Here's how the part is built. I have some questions about the finished solid (model axes, mm). Round coordinates to 2 decimals unless told otherwise and drop trailing zeros. Loops run counter-clockwise (first coordinate to the right, second up) from the corner with the lowest first, then second, coordinate; pieces in that order, holes last. Notation, with made-up numbers: M -30,-9.75 L 23,-9.75 A21 cw 23,9.25 Z; hole C 25.25,57 d11. An arc over 180 degrees is marked long. Put each result on its own line as item: value. Start each with the question number.
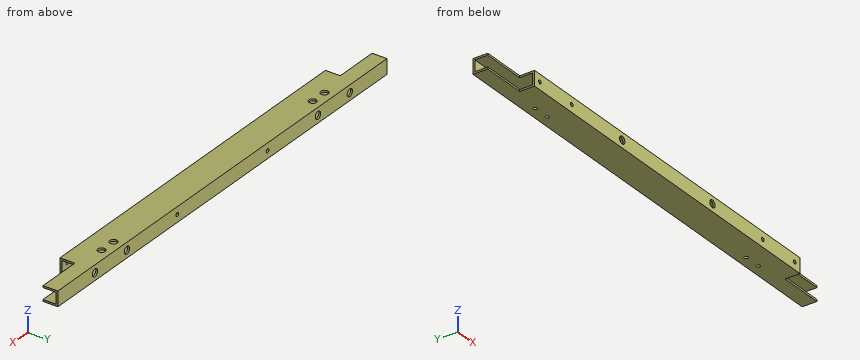
Autodesk Inventor part; units mm, degrees
ref_plane "YZ Plane" through (0, 0, 0) normal (1, 0, 0) x (0, 1, 0)
ref_plane "XZ Plane" through (0, 0, 0) normal (0, 1, 0) x (-1, 0, 0)
ref_plane "XY Plane" through (0, 0, 0) normal (0, 0, 1) x (1, 0, 0)
sketch "Sketch1" plane through (0, 0, 0) normal (0, 0, 1) x (1, 0, 0)
  line L0 (0, 0) -> (787.4, 0)
  line L1 (787.4, 0) -> (787.4, 50.8)
  line L2 (787.4, 50.8) -> (565.5048, 50.8)
  line L3 (565.5048, 50.8) -> (348.1028, 50.8)
  line L4 (348.1028, 50.8) -> (130.7008, 50.8)
  line L5 (130.7008, 50.8) -> (0, 50.8)
  line L6 (0, 50.8) -> (0, 0)
  dimension "d2" = 50.8
  dimension "d3" = 50.8
  dimension "d4" = 787.4
extrude "Extrusion1" add sketch "Sketch1" along normal blind 25.4
shell "Shell1" thickness 3.175 removed faces 2 at (0, 33.8667, 16.9333) at (787.4, 16.9333, 16.9333)
sketch "Sketch2" plane through (0, 0, 25.4) normal (0, 0, 1) x (1, 0, 0)
  line L0 (0, 0) -> (76.2, 0)
  line L1 (76.2, 0) -> (76.2, 25.4)
  line L2 (76.2, 25.4) -> (0, 25.4)
  line L3 (0, 25.4) -> (0, 0)
  line L4 (787.4, 0) -> (711.2, 0)
  line L5 (711.2, 0) -> (711.2, 25.4)
  line L6 (711.2, 25.4) -> (787.4, 25.4)
  line L7 (787.4, 25.4) -> (787.4, 0)
  dimension "d9" = 25.4
  dimension "d12" = 76.2
extrude "Extrusion2" cut sketch "Sketch2" against normal through all
sketch "Sketch4" plane through (0, 50.8, 0) normal (0, 1, 0) x (1, 0, 0)
  line L0 (787.4, 0) -> (787.4, -25.4)
  line L1 (787.4, 0) -> (0, 0)
  circle A0 centre (501.65, -12.7) radius 3.175
  circle A1 centre (285.75, -12.7) radius 3.175
  dimension "d21" = 285.75
  dimension "d22" = 215.9
  dimension "d23" = 12.7
  dimension "d24" = 12.7
  dimension "d25" = 6.35
  dimension "d26" = 6.35
extrude "Extrusion4" cut sketch "Sketch4" against normal through all
sketch "Sketch5" plane through (76.2, 0, 0) normal (0, -1, 0) x (1, 0, 0)
  circle A0 centre (209.55, 12.7) radius 3.175
  circle A1 centre (425.45, 12.7) radius 3.175
  circle A2 centre (209.55, 12.7) radius 6.35
  circle A3 centre (425.45, 12.7) radius 6.35
  point P0 (-76.2, 0)
  dimension "d29" = 12.7
  dimension "d30" = 12.7
extrude "Extrusion5" cut sketch "Sketch5" against normal up to next
sketch "Sketch6" plane through (76.2, 0, 0) normal (0, -1, 0) x (1, 0, 0)
  line L0 (635, 25.4) -> (0, 25.4)
  circle A0 centre (12.6948, 12.7) radius 3.175
  circle A1 centre (88.8948, 12.7) radius 3.175
  circle A2 centre (546.1057, 12.7) radius 3.175
  circle A3 centre (622.3057, 12.7) radius 3.175
  line L1 (711.2, 22.225) -> (711.2, 3.175)
  line L2 (-76.2, 3.175) -> (-76.2, 22.225)
  point P0 (-76.2, 0)
  dimension "d33" = 88.8943
  dimension "d34" = 76.2
  dimension "d35" = 6.35
  dimension "d36" = 12.7
  dimension "d37" = 12.7
  dimension "d38" = 12.7
  dimension "d39" = 12.7
  dimension "d40" = 88.8948
  dimension "d41" = 76.2
extrude "Extrusion6" cut sketch "Sketch6" against normal through all
sketch "Sketch7" plane through (0, 50.8, 0) normal (0, 1, 0) x (1, 0, 0)
  circle A0 centre (698.5057, -12.7) radius 3.175
  circle A1 centre (622.3057, -12.7) radius 3.175
  circle A2 centre (165.0948, -12.7) radius 3.175
  circle A3 centre (88.8948, -12.7) radius 3.175
  circle A4 centre (698.5057, -12.7) radius 6.35
  circle A5 centre (622.3057, -12.7) radius 6.35
  circle A6 centre (88.8948, -12.7) radius 6.35
  circle A7 centre (165.0948, -12.7) radius 6.35
  dimension "d44" = 12.7
extrude "Extrusion7" cut sketch "Sketch7" against normal up to next
sketch "Sketch8" plane through (0, 0, 25.4) normal (0, 0, 1) x (1, 0, 0)
  line L0 (787.4, 50.8) -> (787.4, 25.4)
  line L1 (0, 50.8) -> (787.4, 50.8)
  circle A0 centre (631.825, 34.925) radius 3.175
  circle A1 centre (660.4, 34.925) radius 3.175
  line L2 (631.825, 34.925) -> (660.4, 34.925) construction
  line L3 (0, 25.4) -> (0, 50.8)
  line L4 (631.825, 34.925) -> (155.575, 34.925) construction
  line L5 (155.575, 34.925) -> (127, 34.925) construction
  line L6 (127, 34.925) -> (0, 34.925) construction
  circle A2 centre (127, 34.925) radius 3.175
  circle A3 centre (155.575, 34.925) radius 3.175
  point P0 (0, 0)
  dimension "d47" = 127
  dimension "d48" = 28.575
  dimension "d49" = 15.875
  dimension "d50" = 6.35
  dimension "d53" = 127
  dimension "d54" = 28.575
  dimension "d55" = 476.25
extrude "Extrusion8" cut sketch "Sketch8" against normal through all
sketch "Sketch9" plane through (0, 0, 25.4) normal (0, 0, 1) x (1, 0, 0)
  circle A0 centre (155.575, 34.925) radius 3.175
  circle A1 centre (127, 34.925) radius 3.175
  circle A2 centre (660.4, 34.925) radius 3.175
  circle A3 centre (631.825, 34.925) radius 3.175
  circle A4 centre (631.825, 34.925) radius 6.35
  circle A5 centre (660.4, 34.925) radius 6.35
  circle A6 centre (127, 34.925) radius 6.35
  circle A7 centre (155.575, 34.925) radius 6.35
  point P0 (0, 0)
  dimension "d56" = 12.7
extrude "Extrusion9" cut sketch "Sketch9" against normal up to next
properties part number "FrameRepresentation_FrontRear" material "Aluminum-6061"
1) If I drill on probe 1 along X at (y, z) = (35, 1.75); probe 2 along Y at (x, z) = (365.5, 16.5) (3 decimals); probe 3 along Z at (x, y) = (98.5, 41.5) (3 decimals), over which ranges is the centre line in solid material (lowest first)? Write a range as from..to.
2) Suppose I cut it at B-B (x = 415). Write out the boundary of the cut face in (y, z) (3 decimals), plus the area to 3 significant figures.
3) I'm going to push flat-ended pins straight in: P1, Ø5, axis at x = 155.575, y = 34.925, coming from the +Z side; P2, Ø11.5, axis at x = 622.31, z = 12.7, coming from the +Y side (3 decimals); P3, Ø8.5, axis at x = 501.65, z = 12.7, coming from the -Y side (3 decimals); P4, Ø12.5, axis at y = 14, z = 7.5, coming from the -X side. Where does each tip first touch, or does it pass through?
4) Suppose I cut it at A-A (y = 19). Write out the boundary of the cut face in (x, z) (3 decimals).
Results are:
1. probe 1: 0..123.83, 130.17..152.4, 158.75..628.65, 635..657.23, 663.57..787.4
1. probe 2: 0..3.175, 47.625..50.8
1. probe 3: 0..3.175, 22.225..25.4
2. outline: M 0,0 L 50.8,0 L 50.8,25.4 L 0,25.4 Z; hole M 3.175,3.175 L 47.625,3.175 L 47.625,22.225 L 3.175,22.225 Z
2. area: 444 mm²
3. P1: through
3. P2: y = 3.175
3. P3: y = 47.625
3. P4: x = 76.2
4. outline: M 76.2,0 L 711.2,0 L 711.2,3.175 L 76.2,3.175 Z; M 76.2,22.225 L 711.2,22.225 L 711.2,25.4 L 76.2,25.4 Z
